```python
from build123d import *

# Parameters (mm, degrees)
BOSS_EXTRUDE1_DEPTH     = 15
SKETCH2_R               = 4
CUT_EXTRUDE1_DEPTH      = 10
LPATTERN1_COUNT         = 3
LPATTERN1_PITCH         = 142
SKETCH3_R               = 4
CUT_EXTRUDE2_DEPTH      = 10
LPATTERN2_COUNT         = 2
LPATTERN2_PITCH         = 106
MIRROR1_COPY_1_SKETCH_R = 4
MIRROR1_COPY_1_DEPTH    = 10
SKETCH4_W               = 400
SKETCH4_H               = 15
BOSS_EXTRUDE2_DEPTH     = 15


with BuildPart() as part:
    # Sketch1 → Boss-Extrude1 (new body)
    with BuildSketch(Plane.XY):
        Polygon((-200, -75.5), (-200, -85.5), (200, -85.5), (200, -75.5), (200, 75.5), (-200, 75.5), align=None)
    extrude(amount=BOSS_EXTRUDE1_DEPTH)

    # Sketch2 → Cut-Extrude1 (cut)
    with BuildSketch(Plane(origin=(0, 0, 0), x_dir=(-1, 0, 0), z_dir=(0, 0, -1))):
        with Locations((-142, -68)):
            Circle(SKETCH2_R)
    cut_extrude1 = extrude(amount=-CUT_EXTRUDE1_DEPTH, mode=Mode.SUBTRACT)

    # LPattern1: Cut-Extrude1 ×3
    with Locations(*[(-i * LPATTERN1_PITCH, 0, 0) for i in range(1, LPATTERN1_COUNT)]):
        add(cut_extrude1, mode=Mode.SUBTRACT)

    # Sketch3 → Cut-Extrude2 (cut)
    with BuildSketch(Plane(origin=(0, 0, 0), x_dir=(-1, 0, 0), z_dir=(0, 0, -1))):
        with Locations((-164.5, 60.5)):
            Circle(SKETCH3_R)
    cut_extrude2 = extrude(amount=-CUT_EXTRUDE2_DEPTH, mode=Mode.SUBTRACT)

    # LPattern2: Cut-Extrude2 ×2
    with Locations(*[(0, -i * LPATTERN2_PITCH, 0) for i in range(1, LPATTERN2_COUNT)]):
        add(cut_extrude2, mode=Mode.SUBTRACT)

    # Mirror1: Cut-Extrude2 across plane
    add(cut_extrude2.mirror(Plane(origin=(0, 0, 0), x_dir=(0, 0, 1), z_dir=(1, 0, 0))), mode=Mode.SUBTRACT)

    # Mirror1 copy 1 sketch → Mirror1 copy 1 (cut)
    with BuildSketch(Plane(origin=(0, -106, 0), x_dir=(1, 0, 0), z_dir=(0, 0, -1))):
        with Locations((-164.5, -60.5)):
            Circle(MIRROR1_COPY_1_SKETCH_R)
    extrude(amount=-MIRROR1_COPY_1_DEPTH, mode=Mode.SUBTRACT)

    # Sketch4 → Boss-Extrude2 (add)
    with BuildSketch(Plane.XY):
        with Locations((0, -93)):
            Rectangle(SKETCH4_W, SKETCH4_H)
    extrude(amount=BOSS_EXTRUDE2_DEPTH)


solid = part.part
```
Could you check a few things on this model? Use its own coordinates, in mm. A direction names the side the tool comes from. Give positions to 0.01 mm unless a question says otherwise; leave off trailing zeros. Write each loop counter-clockwise with the first axis right and the second up, starting at its lowest first coordinate (ties: lowest second). Pieces come first, ordered by that corner, then holes. Notation, with made-up numbers: (74, 51) -> (80, 51) arc R17 cw to (80, 65) -> close; hole circle Ø3 at (55.25, -37). An arc over 180 degrees is marked (long way). Write each question's results on one line, items separated by ' | '.
1. I need wall thicknesses on L1, parallel to Y at x = 164.5, z = 6; L2, parallel to Y at x = 0, z = 6.5. Which ranges of each line are inside material? Lowest first, please.
Check sheet entries:
L1: y = -100.5 to -49.5, -41.5 to 56.5, 64.5 to 75.5 | L2: y = -100.5 to -72, -64 to 75.5
2. I want a section at A-A, the plane x = -142. Write out the boundary of the cut face in (y, z), then the cut area to 3 significant figures.
Check sheet entries:
outline: (-100.5, 0) -> (-72, 0) -> (-72, 10) -> (-64, 10) -> (-64, 0) -> (75.5, 0) -> (75.5, 15) -> (-100.5, 15) -> close | area: 2,560 mm²
3. Will this pin go through, and if not, where does the flat tip stop? pin 1 Ø2.5 at (x, y) = (143.5, -69) entering from -Z.
Check sheet entries:
pin 1: stops at z = 10
4. On a 3-axis mill with a long thin cutter (end or side, diameter ignored), from which of +Z, -Z, +X, -X, +Y, -Y can I reach the whole of each face in a straight line? I mean faces 1 (the flat face through (3, 75.5, 7)), 2 (the flat face through (0, -68, 10)). Say none if no direction works.
Check sheet entries:
face 1: +Z, -Z, +X, -X, +Y | face 2: -Z
5. I want a section at B-B, the plane y = 60.5. Write out the boundary of the cut face in (x, z).
Check sheet entries:
outline: (-200, 0) -> (-168.5, 0) -> (-168.5, 10) -> (-160.5, 10) -> (-160.5, 0) -> (160.5, 0) -> (160.5, 10) -> (168.5, 10) -> (168.5, 0) -> (200, 0) -> (200, 15) -> (-200, 15) -> close
6. If we mould it in two halves opening along Y, with no side actions, what happens to faces 3 (the cylindrical face through (0.867, -71.905, 4.93)), 4 (the flat face through (-3, -100.5, 7)), 5 (the flat face through (-3, -11, 0))? For each: released by +Y, released by -Y, zero draft, split by the parting line, or undercut.
Check sheet entries:
face 3: undercut | face 4: released by -Y | face 5: zero draft
7. I want a section at C-C, the plane y = -68. Write out the boundary of the cut face in (x, z), then the cut area to 3 significant figures.
Check sheet entries:
outline: (-200, 0) -> (-146, 0) -> (-146, 10) -> (-138, 10) -> (-138, 0) -> (-4, 0) -> (-4, 10) -> (4, 10) -> (4, 0) -> (138, 0) -> (138, 10) -> (146, 10) -> (146, 0) -> (200, 0) -> (200, 15) -> (-200, 15) -> close | area: 5,760 mm²
